from build123d import *

# Parameters (mm, degrees)
SKETCH3_W               = 149.929020718
SKETCH3_H               = 96.78
SKETCH3_R               = 2.65
BOSS_EXTRUDE1_DEPTH     = 10
SKETCH4_W               = 30
SKETCH4_H               = 12
BOSS_EXTRUDE4_DEPTH     = 13
CUT_EXTRUDE1_DEPTH      = 116.506286536
CUT_EXTRUDE1_DEPTH_BACK = 116.506286536
SKETCH5_R               = 2.65
FILLET1_R               = 1


with BuildPart() as part:
    # Sketch3 → Boss-Extrude1 (new body)
    with BuildSketch(Plane.XY):
        with Locations((-0.035848502, 4.44)):
            Rectangle(SKETCH3_W, SKETCH3_H)
        with Locations((-53.055358861, -17.005)):
            Circle(SKETCH3_R, mode=Mode.SUBTRACT)
        with Locations((-33.055, -17.005)):
            Circle(SKETCH3_R, mode=Mode.SUBTRACT)
        with Locations((33.055, -17.005)):
            Circle(SKETCH3_R, mode=Mode.SUBTRACT)
        with Locations((53.054641139, -17.005)):
            Circle(SKETCH3_R, mode=Mode.SUBTRACT)
        with Locations((-13.055, 24.027361408)):
            Circle(SKETCH3_R, mode=Mode.SUBTRACT)
        with Locations((13.055, 24.027361408)):
            Circle(SKETCH3_R, mode=Mode.SUBTRACT)
        with Locations((-53.055358861, 25.027361408)):
            Circle(SKETCH3_R, mode=Mode.SUBTRACT)
        with Locations((-33.055, 25.027361408)):
            Circle(SKETCH3_R, mode=Mode.SUBTRACT)
        with Locations((33.055, 25.027361408)):
            Circle(SKETCH3_R, mode=Mode.SUBTRACT)
        with Locations((53.054641139, 25.027361408)):
            Circle(SKETCH3_R, mode=Mode.SUBTRACT)
    extrude(amount=BOSS_EXTRUDE1_DEPTH)

    # Sketch4 → Boss-Extrude4 (add)
    with BuildSketch(Plane.XY.offset(10)):
        with Locations((-33.055, -37.95)):
            Rectangle(SKETCH4_W, SKETCH4_H)
        Polygon((-48.055, 40.83), (-18.055, 40.83), (18.055, 40.83), (48.055, 40.83), (48.055, 52.83), (18.055, 52.83), (-18.055, 52.83), (-48.055, 52.83), align=None)
        with Locations((33.055, -37.95)):
            Rectangle(SKETCH4_W, SKETCH4_H)
    extrude(amount=BOSS_EXTRUDE4_DEPTH)

    # Sketch5 → Cut-Extrude1 (cut, two sides: drawn at the far end of the back side and taken through both)
    with BuildSketch(Plane(origin=(0, -31.95, 0), x_dir=(1, 0, 0), z_dir=(0, 1, 0)).offset(-CUT_EXTRUDE1_DEPTH_BACK)):
        with Locations(Location((33.055, -16.5, 0), (0, 0, 270))):
            Circle(SKETCH5_R)
        with Locations(Location((-33.055, -16.5, 0), (0, 0, 270))):
            Circle(SKETCH5_R)
    extrude(amount=CUT_EXTRUDE1_DEPTH + CUT_EXTRUDE1_DEPTH_BACK, mode=Mode.SUBTRACT)

    # Fillet1
    fillet1_edges = [part.edges().sort_by_distance(p)[0] for p in [
        (-48.055, 46.83, 10),
        (48.055, 46.83, 10),
        (0, 40.83, 10),
        (-18.055, -37.95, 10),
        (-33.055, -31.95, 10),
        (-48.055, -37.95, 10),
        (48.055, -37.95, 10),
        (33.055, -31.95, 10),
        (18.055, -37.95, 10),
    ]]
    fillet(fillet1_edges, radius=FILLET1_R)


solid = part.part
Verification items for the finished model (mm, model axes). A direction names the side the tool comes from. Coordinates: 2 decimals unless noted, no trailing zeros. Order: outer loops, then holes, each group sorted by start corner. A loop starts at its lowest first (then second) coordinate and runs counter-clockwise, first axis right, second up. Notation, with made-up numbers: M 49.25,23.5 L 97.25,23.5 A15 cw 97.25,32.5 Z; hole C 85,84.5 d11. An arc over 180 degrees is marked long. One line per item, written item: value. Start each with the question number.
Item 1: Sectioned sample at B-B on x = -53. Record the cut outline in (y, z).
Item 2: Sectioned sample at A-A on z = 16.5. Record the cut outline in (x, y) (3 decimals).
Item 3: Sectioned sample at C-C on y = -35. Record the cut outline in (x, z) (3 decimals).
Item 4: Mould release check, pull along Y, two halves, no side actions. Record for faces 1 (the cylindrical face through (55.582, -16.209, 4.93)), 2 (the flat face through (-1, -43.95, 6)), 3 (the flat face through (18.055, -38, 17)): pulls with the +Y half, pulls with the -Y half, needs draft (parallel to the pull), parting line crosses it, or undercut.
Item 5: Sectioned sample at D-D on x = 39.5. Record the cut outline in (y, z), then the cut area to 3 significant figures.
Item 6: Depth check by flat-ended pin: P1, Ø6, axis at y = -38.5, z = 16, coming from the +X side (3 decimals); P2, Ø7, axis at x = -53.06, y = -17, coming from the +Z side; P3, Ø3.5, axis at y = -40.5, z = 17, coming from the -X side (3 decimals). Enter the tip coordinate at first touch or a pass-through.
Item 7: Access from +Z, -Z, +X, -X, +Y, -Y to the whole of each face (thin tool, end or side, straight path). Record for faces 4 (the flat face through (-48.055, -38, 17)), 5 (the flat face through (-18.055, -38, 17)), 6 (the flat face through (48.055, 47, 17)).
Item 8: Thickness scan on probe 1 along X at (y, z) = (46.5, 16.5) (3 decimals); probe 2 along X at (y, z) = (-37, 16.5) (3 decimals); probe 3 along X at (y, z) = (-35.5, 20.5) (3 decimals). Record the ranges inside material, lowest first.
Calculated:
1. outline: M -43.95,0 L -19.65,0 L -19.65,10 L -43.95,10 Z; M -14.36,0 L 22.38,0 L 22.38,10 L -14.36,10 Z; M 27.68,0 L 52.83,0 L 52.83,10 L 27.68,10 Z
2. outline: M -48.055,-43.95 L -35.705,-43.95 L -35.705,-31.95 L -48.055,-31.95 Z; M -48.055,40.83 L -35.705,40.83 L -35.705,52.83 L -48.055,52.83 Z; M -30.405,-43.95 L -18.055,-43.95 L -18.055,-31.95 L -30.405,-31.95 Z; M -30.405,40.83 L 30.405,40.83 L 30.405,52.83 L -30.405,52.83 Z; M 18.055,-43.95 L 30.405,-43.95 L 30.405,-31.95 L 18.055,-31.95 Z; M 35.705,-43.95 L 48.055,-43.95 L 48.055,-31.95 L 35.705,-31.95 Z; M 35.705,40.83 L 48.055,40.83 L 48.055,52.83 L 35.705,52.83 Z
3. outline: M -75,0 L 74.929,0 L 74.929,10 L 49.055,10 A1 cw 48.055,11 L 48.055,23 L 18.055,23 L 18.055,11 A1 cw 17.055,10 L -17.055,10 A1 cw -18.055,11 L -18.055,23 L -48.055,23 L -48.055,11 A1 cw -49.055,10 L -75,10 Z; hole C -33.055,16.5 d5.3; hole C 33.055,16.5 d5.3
4. face 1: undercut
4. face 2: pulls with the -Y half
4. face 3: needs draft
5. outline: M -43.95,0 L 52.83,0 L 52.83,23 L 40.83,23 L 40.83,11 A1 cw 39.83,10 L -30.95,10 A1 cw -31.95,11 L -31.95,23 L -43.95,23 Z
5. area: 1,280 mm^2
6. P1: x = 48.055
6. P2: z = 10
6. P3: x = -48.055
7. face 4: +Z, -X, +Y, -Y
7. face 5: +Z, -Y
7. face 6: +Z, +X, +Y, -Y
8. probe 1: -48.055 to -35.705, -30.405 to 30.405, 35.705 to 48.055
8. probe 2: -48.055 to -35.705, -30.405 to -18.055, 18.055 to 30.405, 35.705 to 48.055
8. probe 3: -48.055 to -18.055, 18.055 to 48.055
